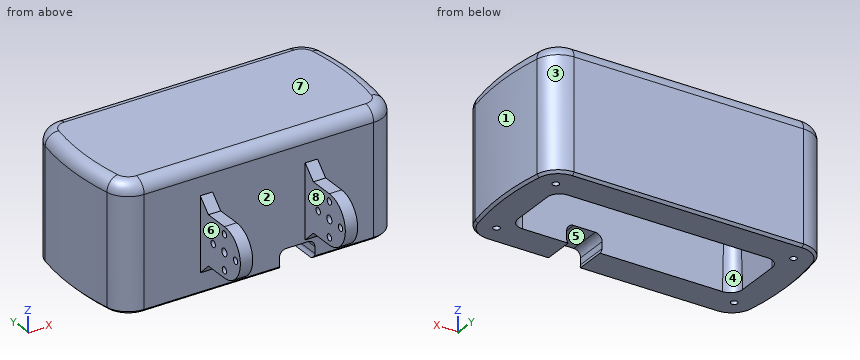
from build123d import *
from OCP.BRepFilletAPI import BRepFilletAPI_MakeChamfer

# Parameters (mm, degrees)
BOSS_EXTRUDE5_DEPTH = 50.8
FILLET9_R           = 5
CHAMFER1_SIZE       = 1
SKETCH8_R           = 1.35
BOSS_EXTRUDE6_DEPTH = 5
CUT_EXTRUDE3_DEPTH  = 20
CHAMFER2_SIZE       = 20
CHAMFER2_SIZE_2     = 0.69841539
SKETCH15_R          = 1.35
CUT_EXTRUDE4_DEPTH  = 5
CUT_EXTRUDE5_REACH  = 96.854


with BuildPart() as part:
    # Sketch2 → Boss-Extrude5 (new body)
    with BuildSketch(Plane.XY):
        with BuildLine():
            Line((46.625, 27.5), (-46.625, 27.5))
            ThreePointArc((-46.625, 27.5), (-53.017219792, 25.190222762), (-56.456518829, 19.327905227))
            ThreePointArc((-56.456518829, 19.327905227), (-58.238005123, 0), (-56.456518829, -19.327905227))
            ThreePointArc((-56.456518829, -19.327905227), (-53.017219792, -25.190222762), (-46.625, -27.5))
            Line((-46.625, -27.5), (46.625, -27.5))
            ThreePointArc((46.625, -27.5), (53.017219792, -25.190222762), (56.456518829, -19.327905227))
            ThreePointArc((56.456518829, -19.327905227), (58.238005123, 0), (56.456518829, 19.327905227))
            ThreePointArc((56.456518829, 19.327905227), (53.017219792, 25.190222762), (46.625, 27.5))
        make_face()
    extrude(amount=BOSS_EXTRUDE5_DEPTH)

    # Fillet9
    fillet9_edges = [part.edges().sort_by_distance(p)[0] for p in [
        (53.017219792, -25.190222762, 50.8),
        (58.238005123, 0, 50.8),
        (53.017219792, 25.190222762, 50.8),
        (0, 27.5, 50.8),
        (-53.017219792, 25.190222762, 50.8),
        (-58.238005123, 0, 50.8),
        (-53.017219792, -25.190222762, 50.8),
        (0, -27.5, 50.8),
    ]]
    fillet(fillet9_edges, radius=FILLET9_R)

    # Chamfer1
    chamfer1_edges = [part.edges().sort_by_distance(p)[0] for p in [
        (58.238005123, 0, 0),
        (53.017219792, -25.190222762, 0),
        (0, -27.5, 0),
        (-53.017219792, -25.190222762, 0),
        (-58.238005123, 0, 0),
        (-53.017219792, 25.190222762, 0),
        (0, 27.5, 0),
        (53.017219792, 25.190222762, 0),
    ]]
    chamfer(chamfer1_edges, length=CHAMFER1_SIZE)

    # Sketch8 → Boss-Extrude6 (add)
    # profile 1 of 2: a face of its own
    with BuildSketch(Plane(origin=(18.825019181, 0, 0), x_dir=(0, 0, -1), z_dir=(1, 0, 0))):
        with BuildLine():
            Line((-13.405087735, -32.61), (-8.405087735, -27.5))
            Line((-8.405087735, -27.5), (-13.405087735, -27.5))
            Line((-13.405087735, -27.5), (-33.413673421, -27.5))
            Line((-33.413673421, -27.5), (-38.413673421, -27.5))
            Line((-38.413673421, -27.5), (-33.405087735, -32.61))
            Line((-33.405087735, -32.61), (-33.405087735, -42.61))
            ThreePointArc((-33.405087735, -42.61), (-23.405087735, -52.61), (-13.405087735, -42.61))
            Line((-13.405087735, -42.61), (-13.405087735, -32.61))
        make_face()
        with BuildLine():
            ThreePointArc((-33.105086536, -42.61), (-23.405087735, -32.910001198), (-13.705088933, -42.61))
            ThreePointArc((-13.705088933, -42.61), (-23.405087735, -52.309998802), (-33.105086536, -42.61))
        make_face(mode=Mode.SUBTRACT)
    # profile 2 of 2: a face of its own
    with BuildSketch(Plane(origin=(18.825019181, 0, 0), x_dir=(0, 0, -1), z_dir=(1, 0, 0))):
        with BuildLine():
            ThreePointArc((-33.105086536, -42.61), (-23.405087735, -52.309998802), (-13.705088933, -42.61))
            ThreePointArc((-13.705088933, -42.61), (-23.405087735, -32.910001198), (-33.105086536, -42.61))
        make_face()
        with Locations((-30.405089608, -42.61)):
            Circle(SKETCH8_R, mode=Mode.SUBTRACT)
        with Locations((-23.405087735, -49.610001873)):
            Circle(SKETCH8_R, mode=Mode.SUBTRACT)
        with Locations((-16.405085862, -42.61)):
            Circle(SKETCH8_R, mode=Mode.SUBTRACT)
        with Locations((-23.405087735, -35.609998127)):
            Circle(SKETCH8_R, mode=Mode.SUBTRACT)
        with BuildLine():
            ThreePointArc((-21.805087735, -42.61), (-23.405087735, -44.21), (-25.005087735, -42.61))
            ThreePointArc((-25.005087735, -42.61), (-23.405087735, -41.01), (-21.805087735, -42.61))
        make_face(mode=Mode.SUBTRACT)
    boss_extrude6 = extrude(amount=BOSS_EXTRUDE6_DEPTH)

    # Mirror1: Boss-Extrude6 across plane
    add(boss_extrude6.mirror(Plane(origin=(0, 0, 0), x_dir=(0, 0, 1), z_dir=(1, 0, 0))))

    # Sketch4 → Cut-Extrude3 (cut)
    with BuildSketch(Plane(origin=(0, 0, 0), x_dir=(-1, 0, 0), z_dir=(0, 0, -1))):
        with BuildLine():
            Line((-40.665, 14.165), (40.665, 14.165))
            ThreePointArc((40.665, 14.165), (44.200533906, 12.700533906), (45.665, 9.165))
            Line((45.665, 9.165), (45.665, -9.165))
            ThreePointArc((45.665, -9.165), (44.200533906, -12.700533906), (40.665, -14.165))
            Line((40.665, -14.165), (-40.665, -14.165))
            ThreePointArc((-40.665, -14.165), (-44.200533906, -12.700533906), (-45.665, -9.165))
            Line((-45.665, -9.165), (-45.665, 9.165))
            ThreePointArc((-45.665, 9.165), (-44.200533906, 12.700533906), (-40.665, 14.165))
        make_face()
    extrude(amount=-CUT_EXTRUDE3_DEPTH, mode=Mode.SUBTRACT)

    # Chamfer2
    chamfer2_edges_1 = [part.edges().sort_by_distance(p)[0] for p in [
        (-45.665, 0, 20),
    ]]
    chamfer2_side_1 = [part.faces().sort_by_distance(p)[0] for p in [
        (-45.665, 0, 19.986031692),
    ]]
    chamfer2_edges_2 = [part.edges().sort_by_distance(p)[0] for p in [
        (-44.200533906, 12.700533906, 20),
    ]]
    chamfer2_side_2 = [part.faces().sort_by_distance(p)[0] for p in [
        (-44.200533906, 12.700533906, 19.986031692),
    ]]
    chamfer2_edges_3 = [part.edges().sort_by_distance(p)[0] for p in [
        (-44.200533906, -12.700533906, 20),
    ]]
    chamfer2_side_3 = [part.faces().sort_by_distance(p)[0] for p in [
        (-44.200533906, -12.700533906, 19.986031692),
    ]]
    chamfer2_edges_4 = [part.edges().sort_by_distance(p)[0] for p in [
        (0, 14.165, 20),
    ]]
    chamfer2_side_4 = [part.faces().sort_by_distance(p)[0] for p in [
        (0, 14.165, 19.986031692),
    ]]
    chamfer2_edges_5 = [part.edges().sort_by_distance(p)[0] for p in [
        (0, -14.165, 20),
    ]]
    chamfer2_side_5 = [part.faces().sort_by_distance(p)[0] for p in [
        (0, -14.165, 19.986031692),
    ]]
    chamfer2_edges_6 = [part.edges().sort_by_distance(p)[0] for p in [
        (44.200533906, 12.700533906, 20),
    ]]
    chamfer2_side_6 = [part.faces().sort_by_distance(p)[0] for p in [
        (44.200533906, 12.700533906, 19.986031692),
    ]]
    chamfer2_edges_7 = [part.edges().sort_by_distance(p)[0] for p in [
        (44.200533906, -12.700533906, 20),
    ]]
    chamfer2_side_7 = [part.faces().sort_by_distance(p)[0] for p in [
        (44.200533906, -12.700533906, 19.986031692),
    ]]
    chamfer2_edges_8 = [part.edges().sort_by_distance(p)[0] for p in [
        (45.665, 0, 20),
    ]]
    chamfer2_side_8 = [part.faces().sort_by_distance(p)[0] for p in [
        (45.665, 0, 19.986031692),
    ]]
    chamfer2 = BRepFilletAPI_MakeChamfer(part.part.solid().wrapped)
    for e in chamfer2_edges_1:
        chamfer2.Add(CHAMFER2_SIZE - 0.0001, CHAMFER2_SIZE_2 - 0.0001, e.wrapped, chamfer2_side_1[0].wrapped)
    for e in chamfer2_edges_2:
        chamfer2.Add(CHAMFER2_SIZE - 0.0001, CHAMFER2_SIZE_2 - 0.0001, e.wrapped, chamfer2_side_2[0].wrapped)
    for e in chamfer2_edges_3:
        chamfer2.Add(CHAMFER2_SIZE - 0.0001, CHAMFER2_SIZE_2 - 0.0001, e.wrapped, chamfer2_side_3[0].wrapped)
    for e in chamfer2_edges_4:
        chamfer2.Add(CHAMFER2_SIZE - 0.0001, CHAMFER2_SIZE_2 - 0.0001, e.wrapped, chamfer2_side_4[0].wrapped)
    for e in chamfer2_edges_5:
        chamfer2.Add(CHAMFER2_SIZE - 0.0001, CHAMFER2_SIZE_2 - 0.0001, e.wrapped, chamfer2_side_5[0].wrapped)
    for e in chamfer2_edges_6:
        chamfer2.Add(CHAMFER2_SIZE - 0.0001, CHAMFER2_SIZE_2 - 0.0001, e.wrapped, chamfer2_side_6[0].wrapped)
    for e in chamfer2_edges_7:
        chamfer2.Add(CHAMFER2_SIZE - 0.0001, CHAMFER2_SIZE_2 - 0.0001, e.wrapped, chamfer2_side_7[0].wrapped)
    for e in chamfer2_edges_8:
        chamfer2.Add(CHAMFER2_SIZE - 0.0001, CHAMFER2_SIZE_2 - 0.0001, e.wrapped, chamfer2_side_8[0].wrapped)
    add(Compound.cast(chamfer2.Shape()), mode=Mode.REPLACE)  # a hair under: the kernel refuses the full size

    # Sketch15 → Cut-Extrude4 (cut)
    with BuildSketch(Plane(origin=(0, 0, 0), x_dir=(-1, 0, 0), z_dir=(0, 0, -1))):
        with Locations((-48.289265859, 18.560867196)):
            Circle(SKETCH15_R)
        with Locations((48.289265859, -18.560867196)):
            Circle(SKETCH15_R)
        with Locations((48.289265859, 18.560867196)):
            Circle(SKETCH15_R)
        with Locations((-48.289265859, -18.560867196)):
            Circle(SKETCH15_R)
    extrude(amount=-CUT_EXTRUDE4_DEPTH, mode=Mode.SUBTRACT)

    # Cut-Extrude5: up to this plane
    cut_extrude5_end = Plane(origin=(-40.665, -13.46658461, 20), z_dir=(0, -0.9993908270190957, 0.03489949670250434))
    # Sketch16 → Cut-Extrude5 (cut, up to the surface)
    with BuildSketch(Plane.XZ.offset(27.5), mode=Mode.PRIVATE) as cut_extrude5_sk1:
        with BuildLine():
            Line((22.750846484, 1.890469849), (22.750846483, 4.590495435))
            add(Edge.make_bspline(
                [(22.750846483, 4.590495435), (22.750837027, 4.775283781), (22.73248867, 4.957224969), (22.66151422, 5.315785643), (22.607726053, 5.494014537), (22.467223433, 5.831520977), (22.381891407, 5.992459845), (22.178053429, 6.297147896), (22.060014741, 6.4405393), (21.673716049, 6.827867738), (21.361341723, 7.036670346), (20.856309918, 7.246376919), (20.679010973, 7.300348953), (20.318322032, 7.372429863), (20.135714984, 7.390453685), (19.950846484, 7.390469849)],
                knots=[0, 0, 0, 0, 0.125, 0.125, 0.25, 0.25, 0.375, 0.375, 0.5, 0.5, 0.75, 0.75, 0.875, 0.875, 1, 1, 1, 1], degree=3))
            Line((19.950846484, 7.390469849), (11.150820748, 7.390469848))
            add(Edge.make_bspline(
                [(11.150820748, 7.390469848), (10.966031816, 7.390460337), (10.784090112, 7.372112007), (10.425528549, 7.301137677), (10.247300018, 7.247346686), (9.909790791, 7.10684451), (9.748851442, 7.021511102), (9.444163129, 6.81766935), (9.300766879, 6.699636548), (8.913443766, 6.313334984), (8.70464106, 6.000960293), (8.49493761, 5.495929858), (8.440966665, 5.318631956), (8.368886124, 4.957943952), (8.350862583, 4.775337528), (8.350846484, 4.590469849)],
                knots=[0, 0, 0, 0, 0.125, 0.125, 0.25, 0.25, 0.375, 0.375, 0.5, 0.5, 0.75, 0.75, 0.875, 0.875, 1, 1, 1, 1], degree=3))
            Line((8.350846484, 4.590469849), (8.350846484, 1.890444263))
            add(Edge.make_bspline(
                [(8.350846484, 1.890444263), (8.35085594, 1.705655915), (8.369204297, 1.523714726), (8.440178749, 1.16515405), (8.493966917, 0.986925155), (8.634469538, 0.649418711), (8.719801566, 0.488479842), (8.923639547, 0.18379179), (9.041678239, 0.040400386), (9.427976936, -0.346928055), (9.740351265, -0.555730668), (10.245383089, -0.765437205), (10.422682029, -0.819409245), (10.783370941, -0.89149025), (10.965977971, -0.909514153), (11.150846484, -0.909530151)],
                knots=[0, 0, 0, 0, 0.125, 0.125, 0.25, 0.25, 0.375, 0.375, 0.5, 0.5, 0.75, 0.75, 0.875, 0.875, 1, 1, 1, 1], degree=3))
            Line((11.150846484, -0.909530151), (19.950871885, -0.90953015))
            add(Edge.make_bspline(
                [(19.950871885, -0.90953015), (20.135660846, -0.909520763), (20.317602552, -0.891172404), (20.676164116, -0.820198035), (20.854392662, -0.766407072), (21.191901959, -0.625904928), (21.352841334, -0.540571521), (21.657529692, -0.336729764), (21.800925955, -0.218696966), (22.18824912, 0.167604602), (22.397051856, 0.479979307), (22.606755334, 0.985009778), (22.66072629, 1.1623077), (22.732806844, 1.522995721), (22.750830385, 1.705602156), (22.750846484, 1.890469849)],
                knots=[0, 0, 0, 0, 0.125, 0.125, 0.25, 0.25, 0.375, 0.375, 0.5, 0.5, 0.75, 0.75, 0.875, 0.875, 1, 1, 1, 1], degree=3))
        make_face()
    cut_extrude5_tool1 = split(extrude(cut_extrude5_sk1.sketch, amount=-CUT_EXTRUDE5_REACH, mode=Mode.PRIVATE), bisect_by=cut_extrude5_end, keep=Keep.BOTH, mode=Mode.PRIVATE)
    add(cut_extrude5_tool1.solids().sort_by_distance((15.550846, -27.5, 3.240452))[0], mode=Mode.SUBTRACT)


solid = part.part
Input: part model. Units: mm. Frame: model coordinates. Face numbers are marked on the shaded views. A direction names the side the tool comes from. Round coordinates to 2 decimals unless told otherwise and drop trailing zeros. Answer as CSV lines item,"result". Start each with the question number.
(1) First-contact query: pin 1 (5.5 mm diameter, centred on x = 20.5, y = -39, fed in from +Z); pin 2 (5 mm diameter, centred on y = -44, z = 15, fed in from -X) (3 decimals); pin 3 (2.5 mm diameter, centred on x = 48.29, y = 18.56, fed in from -Z); pin 4 (1.9 mm diameter, centred on y = -42.61, z = 23.41, fed in from -X). Flat tips, straight axial feed; report the tip coordinate or a pass-through.
(2) Reachability of the marked faces 5, 6, 7 and 8 from +Z, -Z, +X, -X, +Y, -Y: full face, straight path, thin tool, end or side. Return the list, or none.
(3) Line query: line 1 (X direction, y = -34, z = 17); line 2 (Z direction, x = -49, y = -18); line 3 (Z direction, x = 20, y = -42). Output: solid intervals per line, ascending. Write a range as [from, to].
(4) Section A-A, the plane x = -21. State how many separate pieces and enclosed holes the cut face has, plus the area to 3 significant figures.
(5) Draft query along Y for the marked faces 1, 2, 3 and 4. Return one class per face: released by +Y, released by -Y, zero draft, split by the parting line, or undercut.
Values found:
1,pin 1,"stops at z = 33.41"
1,pin 2,"stops at x = -23.825"
1,pin 3,"stops at z = 5"
1,pin 4,"passes through"
2,face 5,"-Z, -Y"
2,face 6,"+Z, -Z, -X, -Y"
2,face 7,"+Z, +X, -X, +Y, -Y"
2,face 8,"+Z, -Z, -Y"
3,line 1,"x = [-23.83, -18.83], [18.83, 23.83]"
3,line 2,"z = [5, 50.8]"
3,line 3,"z = [13.41, 15.2], [17.61, 21.93], [24.88, 29.2], [31.61, 33.41]"
4,separate pieces,"1"
4,enclosed holes,"5"
4,area,"2,680 mm²"
5,face 1,"split by the parting line"
5,face 2,"released by -Y"
5,face 3,"released by +Y"
5,face 4,"undercut"
